Geometry: final body of the model. Coordinates: model frame, mm. Face numbers are marked on the shaded views. A direction names the side the tool comes from. Give positions to 0.01 mm unless a question says otherwise; leave off trailing zeros. Write each loop counter-clockwise with the first axis right and the second up, starting at its lowest first coordinate (ties: lowest second). Pieces come first, ordered by that corner, then holes. Notation, with made-up numbers: (9.5, -23.5) -> (45.5, -23.5) arc R20 ccw to (45.5, -18.5) -> close; hole circle Ø2 at (-4.5, 26.5). An arc over 180 degrees is marked (long way). Answer in a Markdown table with one row per item. Add a question column.
Item 1: Material intervals for probe 1 along X at (y, z) = (0, -4.05); probe 2 along Z at (x, y) = (14, -13.5); probe 3 along X at (y, z) = (0, -6.7), sorted ascending. Write a range as from..to.
Item 2: Section query C-C on y = 17. Output: boundary loops of the cut face in (x, z), plus the area to 3 significant figures.
Item 3: Draft query along Y for the marked faces 1, 2 and 3. Return one class per face: +Y half, -Y half, draft (parallel to the pull), parting line (faces both ways), or undercut.
Item 4: First-contact query: P1, Ø2, axis at x = 10, z = -3.5, coming from the +Y side; P2, Ø1.5, axis at y = 7, z = -7, coming from the +X side; P3, Ø12, axis at x = 10.5, y = -9.5, coming from the -Z side; P4, Ø4, axis at y = -13, z = -1.5, coming from the +X side. Flat tips, straight axial feed; report the tip coordinate or a pass-through.
Item 5: Section query A-A on x = 0. Output: boundary loops of the cut face in (y, z), plus the area to 3 significant figures.
Item 6: Section query D-D on z = -1.5. Output: boundary loops of the cut face in (x, y).
Item 7: Access query for the marked faces 4, 5 and 6. Directions: +Z, -Z, +X, -X, +Y, -Y. A direction counts if a zero-diameter tool reaches every point of the face in a straight line with its end or side. Return the directions, or none.
Item 8: Section query B-B on z = -5.75. Output: boundary loops of the cut face in (x, y).
```python
from build123d import *

# Parameters (mm, degrees)
CUT_EXTRUDE_1_DEPTH      = 11
CUT_EXTRUDE_1_DEPTH_BACK = 3
CUT_EXTRUDE_2_DEPTH      = 21


with BuildPart() as part:
    # Эскиз1 → Повернуть1 (revolve)
    with BuildSketch(Plane(origin=(0, 0, 0), x_dir=(0, 0, -1), z_dir=(1, 0, 0))):
        Polygon((2.598076211, 13), (5, 13), (5, 14), (9.16435909, 14), (12, 14.5), (12, 20), (10, 20), (10, 16), (0, 16), (0, 14.5), align=None)
    revolve(axis=Axis((0, 0, 0), (0, 0, -1)))

    # Эскиз2 → Вырез-Вытянуть1 (cut, two sides)
    with BuildSketch(Plane.XY.offset(-10)) as cut_extrude_1_sk:
        with BuildLine():
            Line((-16, -12), (-16, 12))
            ThreePointArc((-16, 12), (-20, 0), (-16, -12))
        make_face()
        with BuildLine():
            ThreePointArc((20, 0), (18.973665961, 6.32455532), (16, 12))
            Line((16, 12), (16, -12))
            ThreePointArc((16, -12), (18.973665961, -6.32455532), (20, 0))
        make_face()
    extrude(amount=CUT_EXTRUDE_1_DEPTH, mode=Mode.SUBTRACT)
    extrude(cut_extrude_1_sk.sketch, amount=-CUT_EXTRUDE_1_DEPTH_BACK, mode=Mode.SUBTRACT)

    # Эскиз3 → Вырез-Вытянуть2 (cut, through all)
    with BuildSketch(Plane(origin=(0, 0, 0), x_dir=(1, 0, 0), z_dir=(0, 1, 0))):
        with BuildLine():
            Line((-53.249204779, -27.319040473), (-3.872983346, 0))
            ThreePointArc((-3.872983346, 0), (0, 1), (3.872983346, 0))
            Line((3.872983346, 0), (53.249204779, -27.319040473))
            Line((53.249204779, -27.319040473), (53.249204779, -140.178975177))
            Line((53.249204779, -140.178975177), (-53.249204779, -140.178975177))
            Line((-53.249204779, -140.178975177), (-53.249204779, -27.319040473))
        make_face()
    extrude(amount=CUT_EXTRUDE_2_DEPTH, mode=Mode.SUBTRACT)


solid = part.part
```
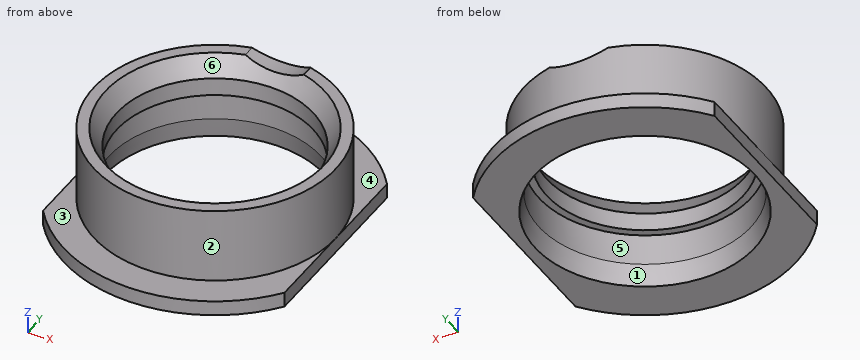
Findings below:
| question | item | result |
|---|---|---|
| 1 | probe 1 | x = -16..-13, 13..16 |
| 1 | probe 2 | z = -12..-10 |
| 1 | probe 3 | x = -16..-14, 14..16 |
| 2 | outline | (-10.54, -12) -> (10.54, -12) -> (10.54, -10) -> (-10.54, -10) -> close |
| 2 | area | 42.1 mm^2 |
| 3 | face 1 | undercut |
| 3 | face 2 | parting line |
| 3 | face 3 | draft |
| 4 | P1 | stops at y = 13.23 |
| 4 | P2 | stops at x = 14.73 |
| 4 | P3 | stops at z = -12 |
| 4 | P4 | stops at x = 11.62 |
| 5 | outline | (-20, -12) -> (-14.5, -12) -> (-14, -9.16) -> (-14, -5) -> (-13, -5) -> (-13, -2.6) -> (-14.5, 0) -> (-16, 0) -> (-16, -10) -> (-20, -10) -> close; (13, -5) -> (14, -5) -> (14, -9.16) -> (14.5, -12) -> (20, -12) -> (20, -10) -> (16, -10) -> (16, -1) -> (13.92, -1) -> (13, -2.6) -> close |
| 5 | area | 66.9 mm^2 |
| 6 | outline | circle Ø32 at (0, 0); hole circle Ø27.27 at (0, 0) |
| 7 | face 4 | +Z, +Y |
| 7 | face 5 | -Z |
| 7 | face 6 | +Z |
| 8 | outline | circle Ø32 at (0, 0); hole circle Ø28 at (0, 0) |
